Verification items for the finished model (mm, model axes). A direction names the side the tool comes from. Round coordinates to 2 decimals unless told otherwise and drop trailing zeros. Write each loop counter-clockwise with the first axis right and the second up, starting at its lowest first coordinate (ties: lowest second). Pieces come first, ordered by that corner, then holes. Notation, with made-up numbers: M 1,15.5 L 41,15.5 A24 cw 41,43.5 Z; hole C 81,68.25 d1. An arc over 180 degrees is marked long. One line per question, with ' | ' between items. Start each with the question number.
Q1. Cross-section at C-C (x = -2.5). Record the boundary of the cut face in (y, z).
Q2. Cross-section at B-B (x = -5). Record the boundary of the cut face in (y, z).
Q3. Cross-section at A-A (z = -4). Record the boundary of the cut face in (x, y), then the cut area to 3 significant figures.
Q4. Thickness scan on line 1 along Y through (x, z) = (0, -1); line 2 along X through (y, z) = (-0.5, 3.5); line 3 along X through (y, z) = (-6.75, 17). Record the ranges inside material, lowest first. Write a range as from..to.
Q5. Cross-section at D-D (z = 6). Record the boundary of the cut face in (x, y), then the cut area to 3 significant figures.
Q6. Tool access check on faces 1 (the face through (0, -11, 16)), 2 (the face through (7.5, 2, 19)), 3 (the face through (-7.5, 2, 19)). Record the directions out of +Z, -Z, +X, -X, +Y, -Y that give a thin tool (end or side, any length) a straight path to the whole face; none if there is none.
Q7. Gauge pin test, flat ends, axial feed: pin 1 (4 mm diameter, centred on x = -2, z = 7.5, fed in from -Y); pin 2 (5 mm diameter, centred on x = -3.5, y = 4, fed in from +Z); pin 3 (10 mm diameter, centred on x = -5.5, y = 8, fed in from -Z). Record the tip position at first contact, or that the pin passes through.
from build123d import *

# Parameters (mm, degrees)
F0_W     = 12
F0_H     = 20
F1_DEPTH = 12
F2_W     = 17
F2_H     = 23
F2_W_2   = 12
F2_H_2   = 20
F3_DEPTH = 3.8
F4_W     = 7
F4_H     = 0.8
F5_DEPTH = 7
F7_DEPTH = 7.5
F8_R     = 1


with BuildPart() as f1:
    # F0 (on Top) → F1 (new body)
    with BuildSketch(Plane.XY):
        Rectangle(F0_W, F0_H)
    extrude(amount=F1_DEPTH)

    # F2 (on face) → F3 (join)
    with BuildSketch(Plane.XY.offset(12)):
        Rectangle(F2_W, F2_H)
        Rectangle(F2_W_2, F2_H_2, mode=Mode.SUBTRACT)
        Rectangle(F2_W_2, F2_H_2)
    extrude(amount=F3_DEPTH)

    # F4 (on face) → F5 (join)
    with BuildSketch(Plane(origin=(0, 0, 0), x_dir=(1, 0, 0), z_dir=(0, 0, -1))):
        with Locations((0, 9.1)):
            Rectangle(F4_W, F4_H)
        with Locations((0, 1.3)):
            Rectangle(F4_W, F4_H)
    extrude(amount=F5_DEPTH)

    # F6 (on Right) → F7 (join, symmetric)
    with BuildSketch(Plane.YZ):
        Polygon((-11, 15.8), (11, 15.8), (11, 24.8), (-11, 17.8), align=None)
    extrude(amount=F7_DEPTH, both=True)

    # F8
    f8_edges = [f1.edges().sort_by_distance(p)[0] for p in [
        (0, 11, 24.8),
        (-7.5, 0, 21.3),
        (0, -11, 17.8),
        (7.5, 0, 21.3),
    ]]
    fillet(f8_edges, radius=F8_R)


solid = f1.part
Determined:
1) outline: M -11.5,12 L -10,12 L -10,0 L -9.5,0 L -9.5,-7 L -8.7,-7 L -8.7,0 L -1.7,0 L -1.7,-7 L -0.9,-7 L -0.9,0 L 10,0 L 10,12 L 11.5,12 L 11.5,15.8 L 11,15.8 L 11,23.43 A1 ccw 9.7,24.39 L -10.3,18.02 A1 ccw -11,17.07 L -11,15.8 L -11.5,15.8 Z
2) outline: M -11.5,12 L -10,12 L -10,0 L 10,0 L 10,12 L 11.5,12 L 11.5,15.8 L 11,15.8 L 11,23.43 A1 ccw 9.7,24.39 L -10.3,18.02 A1 ccw -11,17.07 L -11,15.8 L -11.5,15.8 Z
3) outline: M -3.5,-9.5 L 3.5,-9.5 L 3.5,-8.7 L -3.5,-8.7 Z; M -3.5,-1.7 L 3.5,-1.7 L 3.5,-0.9 L -3.5,-0.9 Z | area: 11.2 mm²
4) line 1: y = -9.5..-8.7, -1.7..-0.9 | line 2: x = -6..6 | line 3: x = -7.5..7.5
5) outline: M -6,-10 L 6,-10 L 6,10 L -6,10 Z | area: 240 mm²
6) face 1: +Z, +X, -X, -Y | face 2: +Z, +X, +Y, -Y | face 3: +Z, -X, +Y, -Y
7) pin 1: stops at y = -10 | pin 2: stops at z = 23.37 | pin 3: stops at z = 0
